Can you work these out from the model? Positions are in its coordinate system, mm. Round coordinates to 2 decimals unless told otherwise and drop trailing zeros. Loops run counter-clockwise (first coordinate to the right, second up) from the corner with the lowest first, then second, coordinate; pieces in that order, holes last. Notation, with made-up numbers: (-27, -30.5) -> (21, -30.5) arc R23 cw to (21, 6.5) -> close; hole circle Ø8 at (9.25, 37). An arc over 180 degrees is marked (long way). Answer as a JSON object with one key per item and string values.
```python
from build123d import *

# Parameters (mm, degrees)
BOSS_EXTRUDE1_DEPTH = 3.175
SKETCH3_R           = 130.556
CUT_EXTRUDE2_DEPTH  = 4.175
SKETCH4_R           = 8.255
CUT_EXTRUDE3_DEPTH  = 4.175


with BuildPart() as part:
    # Sketch1 → Boss-Extrude1 (new body)
    with BuildSketch(Plane(origin=(0, 0, 0), x_dir=(1, 0, 0), z_dir=(0, 1, 0))):
        Polygon((-205.417689271, 85.086792847), (-205.417689271, -85.086792847), (-85.086792847, -205.417689271), (85.086792847, -205.417689271), (205.417689271, -85.086792847), (205.417689271, 85.086792847), (205.417689271, 135.886792847), (-205.417689271, 135.886792847), align=None)
    extrude(amount=BOSS_EXTRUDE1_DEPTH)

    # Sketch3 → Cut-Extrude2 (cut, through all)
    with BuildSketch(Plane(origin=(0, 3.175, 0), x_dir=(-1, 0, 0), z_dir=(0, 1, 0))):
        with Locations(Location((41.979295667, 41.979295667, 0), (0, 0, 90))):  # turned: the seam where the file's is
            Circle(SKETCH3_R)
    extrude(amount=-CUT_EXTRUDE2_DEPTH, mode=Mode.SUBTRACT)

    # Sketch4 → Cut-Extrude3 (cut, through all)
    with BuildSketch(Plane(origin=(0, 3.175, 0), x_dir=(1, 0, 0), z_dir=(0, 1, 0))):
        with Locations(Location((147.81822682, -27.487330396, 0), (0, 0, 270))):  # turned: the seam where the file's is
            Circle(SKETCH4_R)
    extrude(amount=-CUT_EXTRUDE3_DEPTH, mode=Mode.SUBTRACT)


solid = part.part
```
Q1. We'd pull the mould along Z, two halves only. Please class faces 1 (the cylindrical face through (-169.43, 1.61, 13.68)), 2 (the flat face through (-146.095, 1.565, 144.41)), 3 (the flat face through (88, 3.175, -6)): pulls with the +Z half, pulls with the -Z half, needs draft (parallel to the pull), parting line crosses it, or undercut.
Determined:
{"face 1": "undercut", "face 2": "pulls with the +Z half", "face 3": "needs draft"}
Q2. I want a section at B-B, the plane x = 52. Write out the boundary of the cut face in (y, z) (3 decimals), then the cut area to 3 significant figures.
Determined:
{"outline": "(0, -135.887) -> (3.175, -135.887) -> (3.175, -48.645) -> (0, -48.645) -> close; (0, 132.604) -> (3.175, 132.604) -> (3.175, 205.418) -> (0, 205.418) -> close", "area": "508 mm²"}
Q3. I want a section at A-A, the plane z = 52.5. Write out the boundary of the cut face in (x, y) (3 decimals).
Determined:
{"outline": "(-205.418, 0) -> (-172.111, 0) -> (-172.111, 3.175) -> (-205.418, 3.175) -> close; (88.152, 0) -> (205.418, 0) -> (205.418, 3.175) -> (88.152, 3.175) -> close"}
Q4. I want a section at D-D, the plane x = -180.5. Write out the boundary of the cut face in (y, z) (3 decimals).
Determined:
{"outline": "(0, -135.887) -> (3.175, -135.887) -> (3.175, 110.004) -> (0, 110.004) -> close"}
Q5. I'm going to push flat-ended pins straight in: pin 1 (1.5 mm diameter, centred on x = 116.5, y = 3, fed in from +Z); pin 2 (1 mm diameter, centred on x = 118.5, y = 2, fed in from +Z). Where does each tip first touch, or does it pass through?
Determined:
{"pin 1": "z = 174.75", "pin 2": "z = 172.5"}
Q6. If I drill on L1, parallel to X at y = 1.7, z = 20; L2, parallel to X at y = 1.25, z = 23; L3, parallel to X at y = 1.85, z = -8.5, over which ranges is the centre line in solid material (lowest first)? Write a range as [from, to].
Determined:
{"L1": "[-205.42, -170.67], [86.71, 144.34], [151.29, 205.42]", "L2": "[-205.42, -171.15], [87.19, 140.89], [154.75, 205.42]", "L3": "[-205.42, -162.38], [78.42, 205.42]"}
Q7. I want a section at C-C, the plane y = 0.7. Write out the boundary of the cut face in (x, z) (3 decimals), then the cut area to 3 significant figures.
Determined:
{"outline": "(-205.418, -135.887) -> (205.418, -135.887) -> (205.418, 85.087) -> (85.087, 205.418) -> (-85.087, 205.418) -> (-205.418, 85.087) -> close; hole circle Ø261.112 at (-41.979, 41.979); hole circle Ø16.51 at (147.818, 27.487)", "area": "72,000 mm²"}
